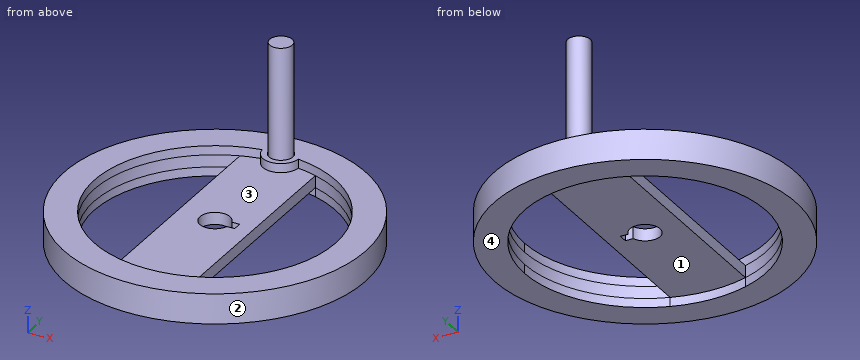
from build123d import *

# Parameters (mm, degrees)
SKETCH_1_R          = 50
EXTRUDE_1_DEPTH     = 5
SKETCH_2_R          = 40
CUT_EXTRUDE_1_DEPTH = 3
CUT_EXTRUDE_2_DEPTH = 10
SKETCH_4_R          = 6
SKETCH_4_R_2        = 4
EXTRUDE_2_DEPTH     = 3
SKETCH_5_R          = 4
CUT_EXTRUDE_3_DEPTH = 3
SKETCH_6_R          = 3.75
EXTRUDE_3_DEPTH     = 40


with BuildPart() as part:
    # Sketch 1 → Extrude 1 (new, symmetric)
    with BuildSketch(Plane.XY):
        Circle(SKETCH_1_R)
        with BuildLine():
            Line((4.769696007, 1.5), (7.369696007, 1.5))
            Line((7.369696007, 1.5), (7.369696007, -1.5))
            Line((7.369696007, -1.5), (4.769696007, -1.5))
            ThreePointArc((4.769696007, -1.5), (-5, 0), (4.769696007, 1.5))
        make_face(mode=Mode.SUBTRACT)
    extrude(amount=EXTRUDE_1_DEPTH, both=True)

    # Sketch 2 → Cut-Extrude 1 (cut)
    with BuildSketch(Plane.XY.offset(5)):
        Circle(SKETCH_2_R)
    cut_extrude_1 = extrude(amount=-CUT_EXTRUDE_1_DEPTH, mode=Mode.SUBTRACT)

    # Mirror 1: Cut-Extrude 1 across plane
    add(cut_extrude_1.mirror(Plane.XY), mode=Mode.SUBTRACT)

    # Sketch 3 → Cut-Extrude 2 (cut)
    with BuildSketch(Plane.XY.offset(2)):
        with BuildLine():
            Line((-12.5, 37.996710384), (-12.5, -37.996710384))
            ThreePointArc((-12.5, -37.996710384), (-40, 0), (-12.5, 37.996710384))
        make_face()
        with BuildLine():
            Line((12.5, 37.996710384), (12.5, -37.996710384))
            ThreePointArc((12.5, -37.996710384), (40, 0), (12.5, 37.996710384))
        make_face()
    extrude(amount=-CUT_EXTRUDE_2_DEPTH, mode=Mode.SUBTRACT)

    # Sketch 5 → Cut-Extrude 3 (cut)
    with BuildSketch(Plane.XY.offset(5)):
        with Locations((0, 40)):
            Circle(SKETCH_5_R)
    extrude(amount=-CUT_EXTRUDE_3_DEPTH, mode=Mode.SUBTRACT)


with BuildPart() as body_2:
    # Sketch 4 → Extrude 2 (new body)
    with BuildSketch(Plane.XY.offset(2)):
        with Locations((0, 40)):
            Circle(SKETCH_4_R)
        with Locations((0, 40)):
            Circle(SKETCH_4_R_2, mode=Mode.SUBTRACT)
    extrude(amount=EXTRUDE_2_DEPTH)


    add(part.part)  # Extrude 3 merges part
    # Sketch 6 → Extrude 3 (add)
    with BuildSketch(Plane.XY.offset(2)):
        with Locations((0, 40)):
            Circle(SKETCH_6_R)
    extrude(amount=EXTRUDE_3_DEPTH)


solid = body_2.part
The model under review builds one solid part; all positions refer to its coordinate system, in mm. Face numbers are marked on the shaded views. Round coordinates to 2 decimals unless told otherwise and drop trailing zeros. Write each loop counter-clockwise with the first axis right and the second up, starting at its lowest first coordinate (ties: lowest second). Pieces come first, ordered by that corner, then holes. Notation, with made-up numbers: M -10.75,84 L 38.25,84 A23 cw 38.25,111 Z; hole C 38.5,65 d1. An arc over 180 degrees is marked long. Answer as CSV lines item,"result". Start each with the question number.
Q1. The part is to be moulded in two halves that separate along Y. For the marked faces 1, 2, 3 and 4, say which applies: +Y half, -Y half, draft (parallel to the pull), parting line (faces both ways), or undercut.
Q2. Consider section D-D, the plane x = 0. Give the boundary of the cut face in (y, z), then the cut area to 3 significant figures.
Q3. Consider section A-A, the plane x = 27. Give the boundary of the cut face in (y, z).
Q4. Consider section B-B, the plane y = 9. Give the boundary of the cut face in (x, z), then the cut area to 3 significant figures.
Q5. Consider section C-C, the plane z = 25. Give the boundary of the cut face in (x, y).
Q6. Wall thickness on line 1 along Y through (x, z) = (0, -0.35); line 2 along X through (y, z) = (34, -1.5); line 3 along Z through (x, y) = (3, 39): over which ranges is each line inside the solid? List them lowest first.
Q7. Clearance check with flat-ended pins moving along their axes: P1, Ø4, axis at x = 11, z = 0.5, coming from the +Y side; P2, Ø10, axis at x = 15.5, y = -4, coming from the +Z side; P3, Ø12.5, axis at x = 1.5, y = 10, coming from the -Z side. State where each tip first meets the part, or that it passes through.
Result set:
1,face 1,"undercut"
1,face 2,"parting line"
1,face 3,"undercut"
1,face 4,"draft"
2,outline,"M -50,-5 L -40,-5 L -40,-2 L -5,-2 L -5,2 L -40,2 L -40,5 L -50,5 Z; M 5,-2 L 40,-2 L 40,-5 L 50,-5 L 50,5 L 44,5 L 44,2 L 43.75,2 L 43.75,42 L 36.25,42 L 36.25,2 L 36,2 L 36,5 L 34,5 L 34,2 L 5,2 Z"
2,area,"774 mm²"
3,outline,"M -42.08,-5 L -29.51,-5 L -29.51,5 L -42.08,5 Z; M 29.51,-5 L 42.08,-5 L 42.08,5 L 29.51,5 Z"
4,outline,"M -49.18,-5 L -38.97,-5 L -38.97,5 L -49.18,5 Z; M -12.5,-2 L 12.5,-2 L 12.5,2 L -12.5,2 Z; M 38.97,-5 L 49.18,-5 L 49.18,5 L 38.97,5 Z"
4,area,"304 mm²"
5,outline,"C 0,40 d7.5"
6,line 1,"y = -50 to -5, 5 to 50"
6,line 2,"x = -36.66 to -21.07, -12.5 to 12.5, 21.07 to 36.66"
6,line 3,"z = -2 to 42"
7,P1,"stops at y = 49.18"
7,P2,"stops at z = 2"
7,P3,"stops at z = -2"
